Answer from the drawing. Dimensions are ordinates in mm from the lowest x, y and z of the part. A direction names the side the tool comes from. Give positions to 0.01 mm unless a question says otherwise; leave off trailing zeros. Write each loop counter-clockwise with the first axis right and the second up, starting at its lowest first coordinate (ties: lowest second). Pieces come first, ordered by that corner, then holes. Notation, with made-up numbers: M -22,53.25 L 16,53.25 A31 cw 16,85.25 Z; hole C 1.5,6.5 d3. An arc over 180 degrees is marked long. Answer as a JSON object with one key per item and string values.
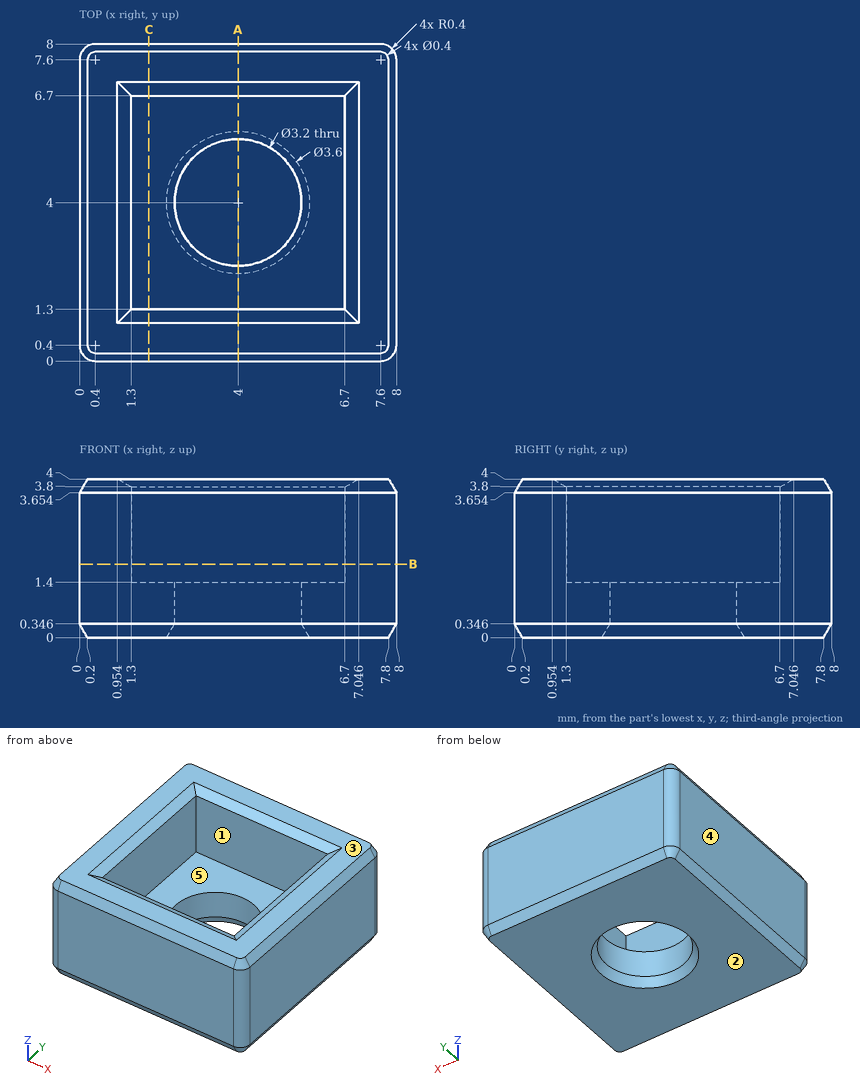
1. A cutting plane is placed at B-B, the plane z = 1.85. Give the vertices of the cut face in (x, y).
Verdict:
{"outline": "M 0,0.4 A0.4 ccw 0.4,0 L 7.6,0 A0.4 ccw 8,0.4 L 8,7.6 A0.4 ccw 7.6,8 L 0.4,8 A0.4 ccw 0,7.6 Z; hole M 1.3,1.3 L 6.7,1.3 L 6.7,6.7 L 1.3,6.7 Z"}
2. A flat-ended cylindrical pin translates along its axis: pin 1 (2 mm diameter, centred on x = 4.5, y = 3.5, fed in from +Z). Find the tip coordinate at first contact, or state that the pin passes through.
Verdict:
{"pin 1": "stops at z = 1.4"}
3. For the marked faces 1 and 2, determine the directions among +Z, -Z, +X, -X, +Y, -Y from which every point of the face is accessible in a straight line to the end or side of a thin tool.
Verdict:
{"face 1": "+Z", "face 2": "-Z, +X, -X, +Y, -Y"}
4. The mould has two halves that part along X. Classify the marked faces 3, 4 and 5: released by +X, released by -X, zero draft, split by the parting line, or undercut.
Verdict:
{"face 3": "zero draft", "face 4": "released by -X", "face 5": "undercut"}
5. A cutting plane is placed at C-C, the plane x = 1.75. Give the vertices of the cut face in (y, z).
Verdict:
{"outline": "M 0,0.35 L 0.2,0 L 7.8,0 L 8,0.35 L 8,3.65 L 7.8,4 L 7.05,4 L 6.7,3.8 L 6.7,1.4 L 1.3,1.4 L 1.3,3.8 L 0.95,4 L 0.2,4 L 0,3.65 Z"}
6. A cutting plane is placed at A-A, the plane x = 4. Give the vertices of the cut face in (y, z).
Verdict:
{"outline": "M 0,0.35 L 0.2,0 L 2.2,0 L 2.4,0.35 L 2.4,1.4 L 1.3,1.4 L 1.3,3.8 L 0.95,4 L 0.2,4 L 0,3.65 Z; M 5.6,0.35 L 5.8,0 L 7.8,0 L 8,0.35 L 8,3.65 L 7.8,4 L 7.05,4 L 6.7,3.8 L 6.7,1.4 L 5.6,1.4 Z"}
7. Consider line 1 along X through (y, z) = (3.5, 3.2); line 2 along X through (y, z) = (4, 0.6). Determine where each line is inside the solid, lowest interval first.
Verdict:
{"line 1": "x = 0 to 1.3, 6.7 to 8", "line 2": "x = 0 to 2.4, 5.6 to 8"}
